from build123d import *

# Parameters (mm, degrees)
SKETCH1_R           = 5.5
BOSS_EXTRUDE1_DEPTH = 3.5
SKETCH2_R           = 5.5
BOSS_EXTRUDE2_DEPTH = 14


with BuildPart() as part:
    # Sketch1 → Boss-Extrude1 (new body)
    with BuildSketch(Plane.XY.offset(300)):
        Polygon((75, 66), (95, 66), (95, -26), (85, -26), (75, -26), (75, 10), (75, 50), (75, 60), align=None)
        with Locations((85, -10)):
            Circle(SKETCH1_R, mode=Mode.SUBTRACT)
        with Locations((85, 50)):
            Circle(SKETCH1_R, mode=Mode.SUBTRACT)
    extrude(amount=BOSS_EXTRUDE1_DEPTH)

    # Sketch2 → Boss-Extrude2 (add)
    with BuildSketch(Plane.XY.offset(303.5)):
        Polygon((75, 10), (75, 85), (75, 95), (95, 95), (95, 66), (95, -26), (75, -26), align=None)
        with Locations((85, 50)):
            Circle(SKETCH2_R, mode=Mode.SUBTRACT)
        with Locations((85, -10)):
            Circle(SKETCH2_R, mode=Mode.SUBTRACT)
    extrude(amount=BOSS_EXTRUDE2_DEPTH)


solid = part.part
Build history of the part. All positions in model axes, mm. A direction names the side the tool comes from. Round coordinates to 2 decimals unless told otherwise and drop trailing zeros. Write each loop counter-clockwise with the first axis right and the second up, starting at its lowest first coordinate (ties: lowest second). Pieces come first, ordered by that corner, then holes. Notation, with made-up numbers: M 71.25,-32 L 92.25,-32 A29 cw 92.25,-10 Z; hole C 79.5,-6 d10. An arc over 180 degrees is marked long. Use CSV: the item, a comma, the result in double quotes.
1. Saw through at B-B (y = 50). Give the cut face in (x, z).
Reply:
outline,"M 75,300 L 79.5,300 L 79.5,317.5 L 75,317.5 Z; M 90.5,300 L 95,300 L 95,317.5 L 90.5,317.5 Z"
2. Two-plate mould, pull along Y, no slides. Class faces 1 (the face through (85, 66, 302)), 2 (the face through (85, 21, 300)), 3 (the face through (85, -26, 309)), 4 (the face through (79.505, -9.758, 308.628)): +Y half, -Y half, draft (parallel to the pull), parting line (faces both ways), or undercut.
Reply:
face 1,"+Y half"
face 2,"draft"
face 3,"-Y half"
face 4,"undercut"
3. Saw through at A-A (x = 85). Give the cut face in (y, z), plus the area to 3 significant figures.
Reply:
outline,"M -26,300 L -15.5,300 L -15.5,317.5 L -26,317.5 Z; M -4.5,300 L 44.5,300 L 44.5,317.5 L -4.5,317.5 Z; M 55.5,300 L 66,300 L 66,303.5 L 95,303.5 L 95,317.5 L 55.5,317.5 Z"
area,"1,630 mm²"
4. Saw through at D-D (x = 92.5). Give the cut face in (y, z), plus the area to 3 significant figures.
Reply:
outline,"M -26,300 L 66,300 L 66,303.5 L 95,303.5 L 95,317.5 L -26,317.5 Z"
area,"2,020 mm²"
5. Wall check: probe 1 along Y at (x, z) = (85, 305.5); probe 2 along Y at (x, z) = (89.5, 316.5); probe 3 along Y at (x, z) = (76.25, 302.75). Give the ranges that are in metal, low to high. Write a range as from..to.
Reply:
probe 1,"y = -26..-15.5, -4.5..44.5, 55.5..95"
probe 2,"y = -26..-13.16, -6.84..46.84, 53.16..95"
probe 3,"y = -26..66"
6. Flat gauge pins, fed straight in: pin 1 (6 mm diameter, centred on x = 89.5, y = 85.5, fed in from -Z); pin 2 (1 mm diameter, centred on x = 80.5, z = 302, fed in from +Y). Where does each tip first touch, or does it go through?
Reply:
pin 1,"stops at z = 303.5"
pin 2,"stops at y = 66"
7. Saw through at C-C (z = 308.5). Give the cut face in (x, y).
Reply:
outline,"M 75,-26 L 95,-26 L 95,95 L 75,95 Z; hole C 85,-10 d11; hole C 85,50 d11"
8. Tool access for faces 5 (the face through (85, 81, 303.5)), 6 (the face through (79.505, 50.242, 308.628)): list every direction of +Z, -Z, +X, -X, +Y, -Y with a clear straight run to the whole face (end or side of a thin tool).
Reply:
face 5,"-Z, +X, -X, +Y"
face 6,"+Z, -Z"
